Work out the finished part from the listing and answer in its coordinate system (mm). A direction names the side the tool comes from. Give positions to 0.01 mm unless a question says otherwise; leave off trailing zeros. Loops run counter-clockwise (first coordinate to the right, second up) from the corner with the lowest first, then second, coordinate; pieces in that order, holes last. Notation, with made-up numbers: (40.25, -32.75) - (49.25, -32.75) arc R18 cw to (49.25, -28.75) - close; hole circle Ø8 at (-2, 45). An arc over 180 degrees is marked (long way). One line per item, written item: value.
from build123d import *

# Parameters (mm, degrees)
BOSS_EXTRU_1_DEPTH           = 10
ENL_V_MAT_EXTRU_1_DEPTH      = 5
ENL_V_MAT_EXTRU_2_DEPTH      = 78.942286341
ENL_V_MAT_EXTRU_2_DEPTH_BACK = 78.942286341
ESQUISSE4_R                  = 5


with BuildPart() as part:
    # Esquisse1 → Boss.-Extru.1 (new body)
    with BuildSketch(Plane.XY):
        Polygon((-32.372583002, 55), (-55, 32.372583002), (-55, -32.372583002), (-32.372583002, -55), (32.372583002, -55), (55, -32.372583002), (55, 32.372583002), (32.372583002, 55), align=None)
    extrude(amount=BOSS_EXTRU_1_DEPTH)

    # Esquisse3 → Enlèv. mat.-Extru.1 (cut)
    with BuildSketch(Plane.XY.offset(10)):
        Polygon((-55, 32.372583002), (-32.372583002, 55), (0, 22.627416998), (32.372583002, 55), (55, 32.372583002), (22.627416998, 0), (55, -32.372583002), (32.372583002, -55), (0, -22.627416998), (-32.372583002, -55), (-55, -32.372583002), (-22.627416998, 0), align=None)
    extrude(amount=-ENL_V_MAT_EXTRU_1_DEPTH, mode=Mode.SUBTRACT)

    # Esquisse4 → Enlèv. mat.-Extru.2 (cut, two sides: drawn at the far end of the back side and taken through both)
    with BuildSketch(Plane.XY.offset(5).offset(-ENL_V_MAT_EXTRU_2_DEPTH_BACK)):
        with Locations((-31.819805153, 31.819805153)):
            Circle(ESQUISSE4_R)
        with Locations((-14.142135624, 14.142135624)):
            Circle(ESQUISSE4_R)
        with Locations((31.819805153, 31.819805153)):
            Circle(ESQUISSE4_R)
        with Locations((14.142135624, 14.142135624)):
            Circle(ESQUISSE4_R)
        with Locations((31.819805153, -31.819805153)):
            Circle(ESQUISSE4_R)
        with Locations((14.142135624, -14.142135624)):
            Circle(ESQUISSE4_R)
        with Locations((-31.819805153, -31.819805153)):
            Circle(ESQUISSE4_R)
        with Locations((-14.142135624, -14.142135624)):
            Circle(ESQUISSE4_R)
        with Locations((0, 38.813708499)):
            Circle(ESQUISSE4_R)
        with Locations((38.813708499, 0)):
            Circle(ESQUISSE4_R)
        with Locations((0, -38.813708499)):
            Circle(ESQUISSE4_R)
        with Locations((-38.813708499, 0)):
            Circle(ESQUISSE4_R)
    extrude(amount=ENL_V_MAT_EXTRU_2_DEPTH + ENL_V_MAT_EXTRU_2_DEPTH_BACK, mode=Mode.SUBTRACT)


solid = part.part
1. Find the intervals of material crossed by line 1 along X through (y, z) = (4.5, 2.5); line 2 along X through (y, z) = (-35, 4.5); line 3 along X through (y, z) = (0, 5.75), in increasing order.
Output:
line 1: x = -55 to -40.99, -36.63 to 36.63, 40.99 to 55
line 2: x = -52.37 to -35.68, -27.96 to -3.23, 3.23 to 27.96, 35.68 to 52.37
line 3: x = -55 to -43.81, -33.81 to -22.63, 22.63 to 33.81, 43.81 to 55
2. For faces 5 (the cylindrical face through (30.74, -36.7, 2.47)), 6 (the flat face through (-39.04, -16.41, 7.54)), determine the directions among +Z, -Z, +X, -X, +Y, -Y from which every point of the face is accessible in a straight line to the end or side of a thin tool.
Output:
face 5: +Z, -Z
face 6: +Z
3. Section B-B (y = 42) is taken. Write down the section's boundary in (x, z).
Output:
outline: (-45.37, 0) - (-3.85, 0) - (-3.85, 10) - (-19.37, 10) - (-19.37, 5) - (-45.37, 5) - close; (3.85, 0) - (45.37, 0) - (45.37, 5) - (19.37, 5) - (19.37, 10) - (3.85, 10) - close
4. The mould has two halves that part along Y. Classify faces 1 (the flat face through (-43.84, -43.53, 2.46)), 2 (the flat face through (0, 55, 5)), 3 (the cylindrical face through (-19.137, -13.922, 2.465)), 4 (the flat face through (55, 0, 5)): released by +Y, released by -Y, zero draft, split by the parting line, or undercut.
Output:
face 1: released by -Y
face 2: released by +Y
face 3: undercut
face 4: zero draft
5. Flat-ended cylindrical pins translate along their axes: pin 1 Ø8 at (x, y) = (-31.82, -31.82) entering from -Z; pin 2 Ø2 at (x, y) = (26.5, -43.5) entering from +Z. Find the tip coordinate at first contact, or state that the pin passes through.
Output:
pin 1: passes through
pin 2: stops at z = 5
6. Section C-C (z = 3) is taken. Count the separate pieces of the cut face and the enclosed holes in it, and give its area (3 significant figures).
Output:
separate pieces: 1
enclosed holes: 12
area: 10,100 mm²
7. Section D-D (y = -17) is taken. Write down the section's boundary in (x, z).
Output:
outline: (-55, 0) - (-18.24, 0) - (-18.24, 5) - (-39.63, 5) - (-39.63, 10) - (-55, 10) - close; (-10.04, 0) - (10.04, 0) - (10.04, 5) - (-10.04, 5) - close; (18.24, 0) - (55, 0) - (55, 10) - (39.63, 10) - (39.63, 5) - (18.24, 5) - close
8. Section A-A (x = 31) is taken. Write down the section's boundary in (y, z), and give its area (3 significant figures).
Output:
outline: (-55, 0) - (-36.75, 0) - (-36.75, 5) - (-53.63, 5) - (-53.63, 10) - (-55, 10) - close; (-26.89, 0) - (26.89, 0) - (26.89, 5) - (8.37, 5) - (8.37, 10) - (-8.37, 10) - (-8.37, 5) - (-26.89, 5) - close; (36.75, 0) - (55, 0) - (55, 10) - (53.63, 10) - (53.63, 5) - (36.75, 5) - close
area: 549 mm²
